```python
from build123d import *

# Parameters (mm, degrees)
SKETCH1_W           = 127
SKETCH1_H           = 19.05
BOSS_EXTRUDE1_DEPTH = 5.08
SKETCH2_R           = 2.54
BOSS_EXTRUDE2_DEPTH = 10.16


with BuildPart() as part:
    # Sketch1 → Boss-Extrude1 (new body)
    with BuildSketch(Plane.XY):
        with Locations((63.5, 9.525)):
            Rectangle(SKETCH1_W, SKETCH1_H)
    extrude(amount=BOSS_EXTRUDE1_DEPTH)

    # Sketch2 → Boss-Extrude2 (add)
    with BuildSketch(Plane(origin=(0, 0, 0), x_dir=(-1, 0, 0), z_dir=(0, 0, -1))):
        with Locations((-109.22, 3.81)):
            Circle(SKETCH2_R)
        with Locations((-78.74, 3.81)):
            Circle(SKETCH2_R)
        with Locations((-48.26, 3.81)):
            Circle(SKETCH2_R)
        with Locations((-17.78, 3.81)):
            Circle(SKETCH2_R)
    extrude(amount=BOSS_EXTRUDE2_DEPTH)


solid = part.part
```
Design review of the part built by this model. Coordinates are the model's own, in mm. A direction names the side the tool comes from. Give positions to 0.01 mm unless a question says otherwise; leave off trailing zeros. Write each loop counter-clockwise with the first axis right and the second up, starting at its lowest first coordinate (ties: lowest second). Pieces come first, ordered by that corner, then holes. Notation, with made-up numbers: (27, -21.75) -> (47, -21.75) arc R27 cw to (47, 1.25) -> close; hole circle Ø6 at (57.5, -29). An arc over 180 degrees is marked (long way). Answer in a Markdown table with one row per item.
(1) Consider section A-A (y = 3.81). State the section outline as (x, z) points.
Results:
| item | result |
|---|---|
| outline | (0, 0) -> (15.24, 0) -> (15.24, -10.16) -> (20.32, -10.16) -> (20.32, 0) -> (45.72, 0) -> (45.72, -10.16) -> (50.8, -10.16) -> (50.8, 0) -> (76.2, 0) -> (76.2, -10.16) -> (81.28, -10.16) -> (81.28, 0) -> (106.68, 0) -> (106.68, -10.16) -> (111.76, -10.16) -> (111.76, 0) -> (127, 0) -> (127, 5.08) -> (0, 5.08) -> close |
(2) To check wall thickness, follow probe 1 along X at (y, z) = (5.5, -3); probe 2 along X at (y, z) = (4.25, -9); probe 3 along Z at (x, y) = (120.5, 7.75). State the ranges of each line that lie inside material, in increasing order.
Results:
| item | result |
|---|---|
| probe 1 | 15.88 to 19.68, 46.36 to 50.16, 76.84 to 80.64, 107.32 to 111.12 |
| probe 2 | 15.28 to 20.28, 45.76 to 50.76, 76.24 to 81.24, 106.72 to 111.72 |
| probe 3 | 0 to 5.08 |
(3) Consider section B-B (x = 17.78). State the section outline as (y, z) points.
Results:
| item | result |
|---|---|
| outline | (0, 0) -> (1.27, 0) -> (1.27, -10.16) -> (6.35, -10.16) -> (6.35, 0) -> (19.05, 0) -> (19.05, 5.08) -> (0, 5.08) -> close |
(4) Clearance check with flat-ended pins moving along their axes: pin 1 (2 mm diameter, centred on x = 44.5, y = 5, fed in from -Z); pin 2 (5 mm diameter, centred on y = 15, z = -4, fed in from +X); pin 3 (6 mm diameter, centred on x = 26, z = -2, fed in from -Y). State where each tip first meets the part, or that it passes through.
Results:
| item | result |
|---|---|
| pin 1 | z = 0 |
| pin 2 | through |
| pin 3 | y = 0 |
(5) For faces 1 (the flat face through (79, 4, -10.16)), 2 (the cylindrical face through (18.11, 6.33, -5.01)), list the 3-axis set-ups (+Z, -Z, +X, -X, +Y, -Y) from which the entire face can be reached by the end or side of a thin tool; tool diameter is ignored.
Results:
| item | result |
|---|---|
| face 1 | -Z, +X, -X, +Y, -Y |
| face 2 | -Z |
(6) Mouldability with a two-part tool opening along X and no side actions: class faces 3 (the cylindrical face through (81.278, 3.922, -5.009)), 4 (the flat face through (63, 10, 5.08)), 5 (the flat face through (0, 9, 3)), 6 (the flat face through (127, 9, 3)) as +X half, -X half, draft (parallel to the pull), parting line (faces both ways), or undercut.
Results:
| item | result |
|---|---|
| face 3 | undercut |
| face 4 | draft |
| face 5 | -X half |
| face 6 | +X half |
(7) Consider section C-C (z = -3.5). State the section outline as (x, y) points, then the cut area to 3 significant figures.
Results:
| item | result |
|---|---|
| outline | circle Ø5.08 at (17.78, 3.81); circle Ø5.08 at (48.26, 3.81); circle Ø5.08 at (78.74, 3.81); circle Ø5.08 at (109.22, 3.81) |
| area | 81.1 mm2 |
(8) Consider section D-D (y = 12.25). State the section outline as (x, z) points, then the cut area to 3 significant figures.
Results:
| item | result |
|---|---|
| outline | (0, 0) -> (127, 0) -> (127, 5.08) -> (0, 5.08) -> close |
| area | 645 mm2 |
